Source: CAD feature listing. Evaluate the final solid. Frame: model axes, mm. Face numbers are marked on the shaded views. Round coordinates to 2 decimals unless told otherwise and drop trailing zeros. Loops run counter-clockwise (first coordinate to the right, second up) from the corner with the lowest first, then second, coordinate; pieces in that order, holes last. Notation, with made-up numbers: M 78.5,-23 L 112.5,-23 A27 ccw 112.5,14 Z; hole C 37,42 d8. An arc over 180 degrees is marked long. One line per item, written item: value.
from build123d import *

# Parameters (mm, degrees)
F1_DEPTH = 0.5


with BuildPart() as f1:
    # F0 (on Top) → F1 (new body)
    with BuildSketch(Plane.XY):
        with BuildLine():
            Line((3.166242, 5.001044), (-5.480078, 11.490485))
            Line((-5.480078, 11.490485), (-11.490485, 5.480078))
            Line((-11.490485, 5.480078), (-5.001044, -3.166242))
            ThreePointArc((-5.001044, -3.166242), (-4.256859, -4.585669), (-4, -6.167633))
            Line((-4, -6.167633), (-4, -9))
            ThreePointArc((-4, -9), (-3.12132, -11.12132), (-1, -12))
            Line((-1, -12), (0, -12))
            ThreePointArc((0, -12), (2.12132, -11.12132), (3, -9))
            Line((3, -9), (3, -7.5))
            ThreePointArc((3, -7.5), (2.853553, -7.146447), (2.5, -7))
            Line((2.5, -7), (0, -7))
            Line((0, -7), (0, 0))
            Line((0, 0), (7, 0))
            Line((7, 0), (7, -2.5))
            ThreePointArc((7, -2.5), (7.146447, -2.853553), (7.5, -3))
            Line((7.5, -3), (9, -3))
            ThreePointArc((9, -3), (11.12132, -2.12132), (12, 0))
            Line((12, 0), (12, 1))
            ThreePointArc((12, 1), (11.12132, 3.12132), (9, 4))
            Line((9, 4), (6.167633, 4))
            ThreePointArc((6.167633, 4), (4.585669, 4.256859), (3.166242, 5.001044))
        make_face()
        with BuildLine():
            ThreePointArc((-2.687006, 5.091169), (-2.687006, 2.687006), (-5.091169, 2.687006))
            Line((-5.091169, 2.687006), (-5.798276, 3.394113))
            ThreePointArc((-5.798276, 3.394113), (-5.798276, 5.798276), (-3.394113, 5.798276))
            Line((-3.394113, 5.798276), (-2.687006, 5.091169))
        make_face(mode=Mode.SUBTRACT)
    extrude(amount=F1_DEPTH)


solid = f1.part
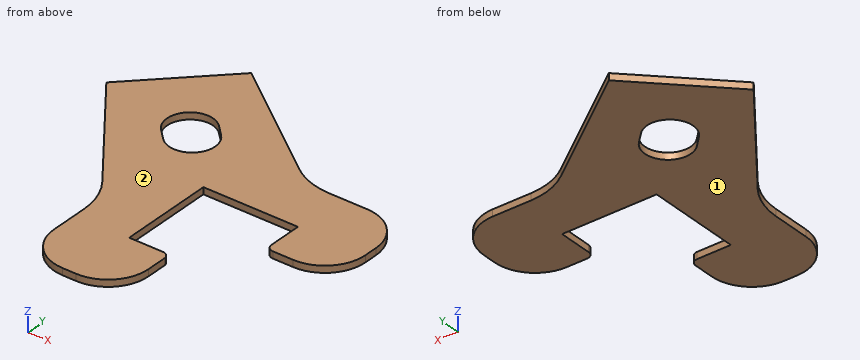
1. Section query D-D (x = 4). Return the cut outline in (y, z).
Report:
outline: M 0,0 L 4.49,0 L 4.49,0.5 L 0,0.5 Z
2. Pin query (flat end, axial travel): pin 1 (1 mm diameter, centred on x = 2, y = -7.5, fed in from -Z). Return the tip coordinate at first contact, or that it passes through.
Report:
pin 1: stops at z = 0
3. Ray query, line 1 (Y direction, x = -6, z = 0.1); line 2 (X direction, y = -1, z = 0.1); line 3 (X direction, y = -2.5, z = 0.15). Return the intervals inside material, ascending. Write a range as [from, to].
Report:
line 1: y = [-1.84, 3.64], [5.56, 10.97]
line 2: x = [-6.63, 0], [7, 11.83]
line 3: x = [-5.5, 0], [7, 10.66]
4. Section query C-C (y = 9). Return the cut outline in (x, z), and give its area (3 significant figures).
Report:
outline: M -7.97,0 L -2.16,0 L -2.16,0.5 L -7.97,0.5 Z
area: 2.90 mm2
5. Section query A-A (z = 0.2). Return the cut outline in (x, y), and give its area (3 significant figures).
Report:
outline: M -11.49,5.48 L -5,-3.17 A5 cw -4,-6.17 L -4,-9 A3 ccw -1,-12 L 0,-12 A3 ccw 3,-9 L 3,-7.5 A0.5 ccw 2.5,-7 L 0,-7 L 0,0 L 7,0 L 7,-2.5 A0.5 ccw 7.5,-3 L 9,-3 A3 ccw 12,0 L 12,1 A3 ccw 9,4 L 6.17,4 A5 cw 3.17,5 L -5.48,11.49 Z; hole M -5.8,3.39 L -5.09,2.69 A1.7 ccw -2.69,5.09 L -3.39,5.8 A1.7 ccw Z
area: 213 mm2
6. Section query B-B (x = 1.5). Return the cut outline in (y, z).
Report:
outline: M -11.6,0 L -7,0 L -7,0.5 L -11.6,0.5 Z; M 0,0 L 6.25,0 L 6.25,0.5 L 0,0.5 Z
7. Pull-direction query (Z, two-part tool) for the marked faces 1 and 2; classes: released by +Z, released by -Z, zero draft, split by the parting line, or undercut.
Report:
face 1: released by -Z
face 2: released by +Z
